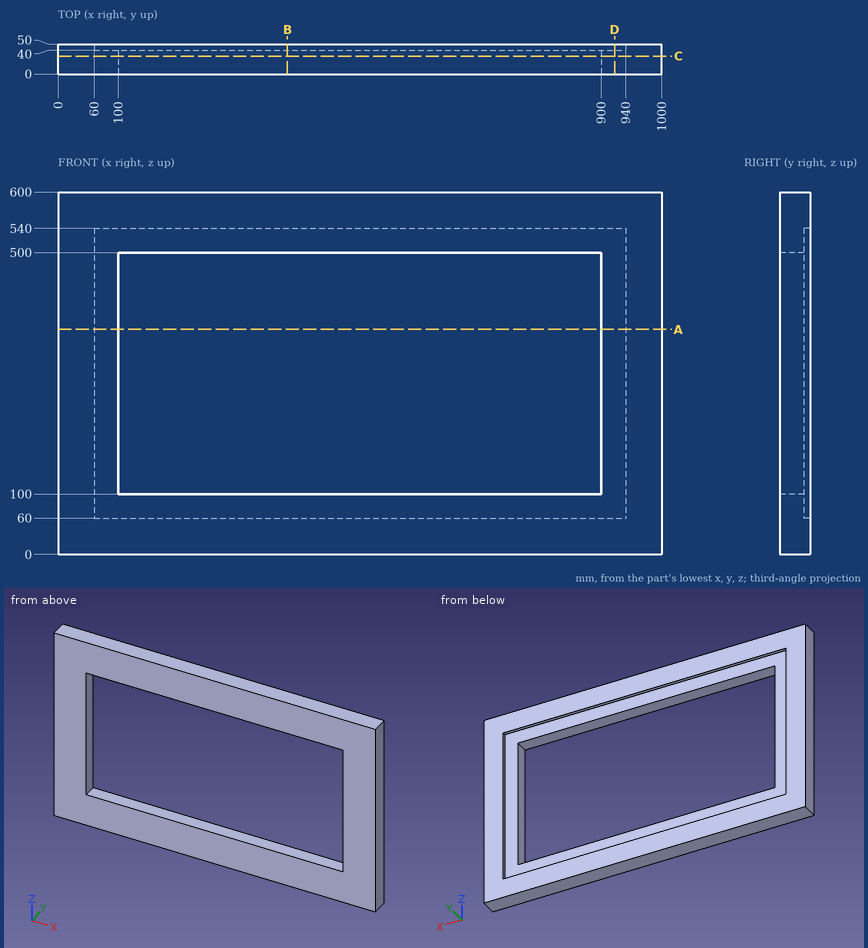
Could you check a few things on this drawing? It's one solid part, dimensions in mm from its lowest x, y, z. Round coordinates to 2 decimals unless told otherwise and drop trailing zeros. Order: outer loops, then holes, each group sorted by start corner. A loop starts at its lowest first (then second) coordinate and runs counter-clockwise, first axis right, second up. Notation, with made-up numbers: M 88,74.25 L 128,74.25 A22 ccw 128,99.25 Z; hole C -24.75,-16 d9. An arc over 180 degrees is marked long. Return JSON: item names as keys, results as strings. Group by question number.
1. If we section it at D-D on x = 922: List the corners of the cut face in (y, z) for me.
2. If we section it at B-B on x = 380: List the corners of the cut face in (y, z) for me, then the cut area to 3 significant figures.
3. If we section it at A-A on z = 373: List the corners of the cut face in (x, y) for me.
4. Please list where these lines run through material, in increasing order: probe 1 along Z at (x, y) = (834, 33); probe 2 along X at (y, z) = (35.5, 341.5); probe 3 along X at (y, z) = (45.5, 98).
5. If we section it at C-C on y = 30: List the corners of the cut face in (x, z) for me, then the cut area to 3 significant figures.
Reply:
{
 "1": {"outline": "M 0,0 L 50,0 L 50,60 L 40,60 L 40,540 L 50,540 L 50,600 L 0,600 Z"},
 "2": {"outline": "M 0,0 L 50,0 L 50,60 L 40,60 L 40,100 L 0,100 Z; M 0,500 L 40,500 L 40,540 L 50,540 L 50,600 L 0,600 Z", "area": "9,200 mm^2"},
 "3": {"outline": "M 0,0 L 100,0 L 100,40 L 60,40 L 60,50 L 0,50 Z; M 900,0 L 1000,0 L 1000,50 L 940,50 L 940,40 L 900,40 Z"},
 "4": {"probe 1": "0 to 100, 500 to 600", "probe 2": "0 to 100, 900 to 1000", "probe 3": "0 to 60, 940 to 1000"},
 "5": {"outline": "M 0,0 L 1000,0 L 1000,600 L 0,600 Z; hole M 100,100 L 900,100 L 900,500 L 100,500 Z", "area": "280,000 mm^2"}
}
